Autodesk Fusion 360 part; units mm, degrees
sketch "Sketch1" plane through (0, 0, 0) normal (0, 1, 0) x (1, 0, 0)
  line L0 (47.5, -22.5) -> (-47.5, -22.5)
  line L1 (-47.5, -22.5) -> (-47.5, 22.5)
  line L2 (-47.5, 22.5) -> (47.5, 22.5)
  line L3 (47.5, 22.5) -> (47.5, -22.5)
  line L4 (47.5, -22.5) -> (-47.5, 22.5) construction
  line L5 (-47.5, -22.5) -> (47.5, 22.5) construction
  line L6 (20, -20) -> (-20, -20)
  line L7 (-20, -20) -> (-20, 20)
  line L8 (-20, 20) -> (20, 20)
  line L9 (20, 20) -> (20, -20)
  line L10 (20, -20) -> (-20, 20) construction
  line L11 (-20, -20) -> (20, 20) construction
  point P0 (-41, 0)
  point P1 (41, 0)
  dimension "d1" = 95
  dimension "d2" = 45
  dimension "d3" = 82
  dimension "d4" = 41
  dimension "d11" = 40
  dimension "d12" = 40
extrude "Extrude1" add sketch "Sketch1" against normal blind 6 contours L0 L1 L2 L3 | L6 L7 L8 L9
hole "Hole1" at (-41, 0, 0) at (41, 0, 0) direction (0, -1, 0) diameter 3.4 depth 35 tip angle 118 counterbore diameter 6.5 counterbore depth 3
extrude "Extrude2" add sketch "Sketch1" along normal blind 40 contours L6 L7 L8 L9
fillet "Fillet1" radius 20 2 edges at (-47.5, -3, 22.5) (-47.5, -3, -22.5)
fillet "Fillet1" radius 20 2 edges at (47.5, -3, 22.5) (47.5, -3, -22.5)
sketch "Sketch2" plane through (0, 0, 20) normal (0, 0, 1) x (1, 0, 0)
  line L0 (-20, 0) -> (20, 0)
  line L1 (20, 0) -> (20, 40)
  line L2 (20, 40) -> (-20, 40)
  line L3 (-20, 40) -> (-20, 0)
  point P0 (-10, 30)
  point P1 (10, 30)
  point P2 (10, 10)
  point P3 (-10, 10)
hole "Hole2" at (10, 30, 20) at (-10, 30, 20) at (-10, 10, 20) at (10, 10, 20) direction (0, 0, -1) diameter 3.4 depth 44 tip angle 118
equation "d4 = d3 / 2"
Source: CAD feature listing. Evaluate the final solid. Frame: model axes, mm. A direction names the side the tool comes from. Give positions to 0.01 mm unless a question says otherwise; leave off trailing zeros. Write each loop counter-clockwise with the first axis right and the second up, starting at its lowest first coordinate (ties: lowest second). Pieces come first, ordered by that corner, then holes. Notation, with made-up numbers: M 41.5,62.25 L 88.5,62.25 A17 cw 88.5,75.25 Z; hole C -17.75,13.25 d3. An arc over 180 degrees is marked long. Return JSON: item names as keys, results as strings. Group by question number.
1) Cut plane C-C, the plane x = -41. Output: boundary loops of the cut face in (y, z).
2) Pin query (flat end, axial travel): P1, Ø4, axis at x = -41, z = 0, coming from the -Y side; P2, Ø3, axis at y = 23, z = 12, coming from the -X side; P3, Ø10, axis at x = -8.5, y = 15, coming from the -Z side; P4, Ø12, axis at y = 11, z = -9.5, coming from the +X side. Return the tip coordinate at first contact, or that it passes through.
3) Cut plane B-B, the plane y = 30. Output: boundary loops of the cut face in (x, z).
4) Cut plane D-D, the plane z = -11.5. Output: boundary loops of the cut face in (x, y), plus the area to 3 significant figures.
5) Material intervals for line 1 along X through (y, z) = (30, 7); line 2 along Y through (x, z) = (-10, 0); line 3 along X through (y, z) = (-2.25, 0), sorted ascending. Write a range as [from, to].
6) Set-up query: faces 1 (the face through (-20, 20, 0)), 2 (the face through (-1, -6, 0)), 3 (the face through (20, 20, 0)), 4 (the face through (44.173, -1.521, -0.705)). Return all of +Z, -Z, +X, -X, +Y, -Y with unobstructed straight access to the full face (end or side cutting, diameter ignored); none if empty.
7) Pull-direction query (X, two-part tool) for faces 5 (the face through (0, 20, -20)), 6 (the face through (10.65, 28.43, -0.28)), 7 (the face through (-41.797, -3.042, -16.486)), 8 (the face through (42.66, -4.52, -0.37)); classes: pulls with the +X half, pulls with the -X half, needs draft (parallel to the pull), parting line crosses it, or undercut.
8) Cut plane A-A, the plane x = 10. Output: boundary loops of the cut face in (y, z), plus the area to 3 significant figures.
Recorded:
{
 "1": {"outline": "M -6,-17.26 L 0,-17.26 L 0,-3.25 L -3,-3.25 L -3,-1.7 L -6,-1.7 Z; M -6,1.7 L -3,1.7 L -3,3.25 L 0,3.25 L 0,17.26 L -6,17.26 Z"},
 "2": {"P1": "stops at y = -6", "P2": "stops at x = -20", "P3": "stops at z = -20", "P4": "stops at x = 20"},
 "3": {"outline": "M -20,-20 L -11.7,-20 L -11.7,20 L -20,20 Z; M -8.3,-20 L 8.3,-20 L 8.3,20 L -8.3,20 Z; M 11.7,-20 L 20,-20 L 20,20 L 11.7,20 Z"},
 "4": {"outline": "M -45.36,-6 L 45.36,-6 L 45.36,0 L 20,0 L 20,40 L -20,40 L -20,0 L -45.36,0 Z; hole C -10,10 d3.4; hole C -10,30 d3.4; hole C 10,10 d3.4; hole C 10,30 d3.4", "area": "2,110 mm²"},
 "5": {"line 1": "x = [-20, -11.7], [-8.3, 8.3], [11.7, 20]", "line 2": "y = [-6, 8.3], [11.7, 28.3], [31.7, 40]", "line 3": "x = [-47.5, -44.25], [-37.75, 37.75], [44.25, 47.5]"},
 "6": {"face 1": "+Z, -Z, -X, +Y", "face 2": "+Z, -Z, +X, -X, -Y", "face 3": "+Z, -Z, +X, +Y", "face 4": "+Y"},
 "7": {"face 5": "needs draft", "face 6": "undercut", "face 7": "pulls with the -X half", "face 8": "undercut"},
 "8": {"outline": "M -6,-22.5 L 0,-22.5 L 0,-20 L 8.3,-20 L 8.3,20 L 0,20 L 0,22.5 L -6,22.5 Z; M 11.7,-20 L 28.3,-20 L 28.3,20 L 11.7,20 Z; M 31.7,-20 L 40,-20 L 40,20 L 31.7,20 Z", "area": "1,600 mm²"}
}
